Source: CAD feature listing. Evaluate the final solid. Frame: model axes, mm. Face numbers are marked on the shaded views. A direction names the side the tool comes from. Give positions to 0.01 mm unless a question says otherwise; leave off trailing zeros. Write each loop counter-clockwise with the first axis right and the second up, starting at its lowest first coordinate (ties: lowest second). Pieces come first, ordered by that corner, then holes. Notation, with made-up numbers: (-36.75, 29) -> (-6.75, 29) arc R18 cw to (-6.75, 54) -> close; hole circle Ø4 at (5.25, 21.5). An arc over 180 degrees is marked (long way). Write item = value, one per line.
from build123d import *

# Parameters (mm, degrees)
BOSS_EXTRUDE1_DEPTH = 2
BOSS_EXTRUDE2_DEPTH = 5
BOSS_EXTRUDE3_DEPTH = 1.5
FILLET1_R           = 2
CUT_EXTRUDE1_DEPTH  = 0.5


with BuildPart() as part:
    # Sketch1 → Boss-Extrude1 (new body)
    with BuildSketch(Plane(origin=(0, 0, 0), x_dir=(1, 0, 0), z_dir=(0, 1, 0))):
        with BuildLine():
            Line((-7.75, -13.25), (7.75, -13.25))
            ThreePointArc((7.75, -13.25), (9.871320344, -12.371320344), (10.75, -10.25))
            Line((10.75, -10.25), (10.75, 10.25))
            ThreePointArc((10.75, 10.25), (9.871320344, 12.371320344), (7.75, 13.25))
            Line((7.75, 13.25), (-7.75, 13.25))
            ThreePointArc((-7.75, 13.25), (-9.871320344, 12.371320344), (-10.75, 10.25))
            Line((-10.75, 10.25), (-10.75, -10.25))
            ThreePointArc((-10.75, -10.25), (-9.871320344, -12.371320344), (-7.75, -13.25))
        make_face()
    extrude(amount=BOSS_EXTRUDE1_DEPTH)

    # Sketch2 → Boss-Extrude2 (add)
    with BuildSketch(Plane(origin=(0, 2, 0), x_dir=(1, 0, 0), z_dir=(0, 1, 0))):
        with BuildLine():
            Line((-7.75, -13.25), (7.75, -13.25))
            ThreePointArc((7.75, -13.25), (9.871320344, -12.371320344), (10.75, -10.25))
            Line((10.75, -10.25), (10.75, 10.25))
            ThreePointArc((10.75, 10.25), (9.871320344, 12.371320344), (7.75, 13.25))
            Line((7.75, 13.25), (-7.75, 13.25))
            ThreePointArc((-7.75, 13.25), (-9.871320344, 12.371320344), (-10.75, 10.25))
            Line((-10.75, 10.25), (-10.75, -10.25))
            ThreePointArc((-10.75, -10.25), (-9.871320344, -12.371320344), (-7.75, -13.25))
        make_face()
        with BuildLine():
            Line((-7.75, -11.5), (7.75, -11.5))
            ThreePointArc((7.75, -11.5), (8.633883476, -11.133883476), (9, -10.25))
            Line((9, -10.25), (9, 10.25))
            ThreePointArc((9, 10.25), (8.633883476, 11.133883476), (7.75, 11.5))
            Line((7.75, 11.5), (-7.75, 11.5))
            ThreePointArc((-7.75, 11.5), (-8.633883476, 11.133883476), (-9, 10.25))
            Line((-9, 10.25), (-9, -10.25))
            ThreePointArc((-9, -10.25), (-8.633883476, -11.133883476), (-7.75, -11.5))
        make_face(mode=Mode.SUBTRACT)
    extrude(amount=BOSS_EXTRUDE2_DEPTH)

    # Sketch3 → Boss-Extrude3 (add)
    with BuildSketch(Plane(origin=(0, 2, 0), x_dir=(1, 0, 0), z_dir=(0, 1, 0))):
        with BuildLine():
            Line((9, -10.25), (-5.75, -10.25))
            ThreePointArc((-5.75, -10.25), (-7.164213562, -9.664213562), (-7.75, -8.25))
            Line((-7.75, -8.25), (-7.75, 8.25))
            ThreePointArc((-7.75, 8.25), (-7.164213562, 9.664213562), (-5.75, 10.25))
            Line((-5.75, 10.25), (9, 10.25))
            Line((9, 10.25), (9, 12.25))
            Line((9, 12.25), (-9.75, 12.25))
            Line((-9.75, 12.25), (-9.75, -12.25))
            Line((-9.75, -12.25), (9, -12.25))
            Line((9, -12.25), (9, -10.25))
        make_face()
    extrude(amount=BOSS_EXTRUDE3_DEPTH)

    # Fillet1
    fillet1_edges = [part.edges().sort_by_distance(p)[0] for p in [
        (0, 0, 13.25),
        (-9.871320344, 0, 12.371320344),
        (-10.75, 0, 0),
        (-9.871320344, 0, -12.371320344),
        (0, 0, -13.25),
        (9.871320344, 0, -12.371320344),
        (10.75, 0, 0),
        (9.871320344, 0, 12.371320344),
    ]]
    fillet(fillet1_edges, radius=FILLET1_R)

    # Sketch4 → Cut-Extrude1 (cut)
    with BuildSketch(Plane(origin=(0, 7, 0), x_dir=(1, 0, 0), z_dir=(0, 1, 0))):
        with BuildLine():
            Line((-7.75, 12.375), (7.75, 12.375))
            ThreePointArc((7.75, 12.375), (9.25260191, 11.75260191), (9.875, 10.25))
            Line((9.875, 10.25), (9.875, -10.25))
            ThreePointArc((9.875, -10.25), (9.25260191, -11.75260191), (7.75, -12.375))
            Line((7.75, -12.375), (-7.75, -12.375))
            ThreePointArc((-7.75, -12.375), (-9.25260191, -11.75260191), (-9.875, -10.25))
            Line((-9.875, -10.25), (-9.875, 10.25))
            ThreePointArc((-9.875, 10.25), (-9.25260191, 11.75260191), (-7.75, 12.375))
        make_face()
    extrude(amount=-CUT_EXTRUDE1_DEPTH, mode=Mode.SUBTRACT)


solid = part.part
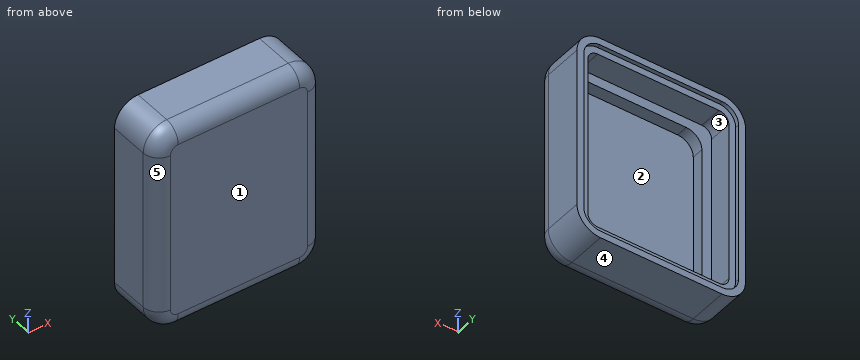
(1) Section query B-B (z = -3). Return loops of the section in (x, y) (3 decimals), plus the area to 3 significant figures.
Values follow:
outline = (-10.75, 2) arc R2 ccw to (-8.75, 0) -> (8.75, 0) arc R2 ccw to (10.75, 2) -> (10.75, 7) -> (9.875, 7) -> (9.875, 6.5) -> (9, 6.5) -> (9, 2) -> (-7.75, 2) -> (-7.75, 3.5) -> (-9, 3.5) -> (-9, 6.5) -> (-9.875, 6.5) -> (-9.875, 7) -> (-10.75, 7) -> close
area = 59.8 mm2
(2) Section query D-D (y = 3). Return loops of the section in (x, z).
Values follow:
outline = (-10.75, -10.25) arc R3 ccw to (-7.75, -13.25) -> (7.75, -13.25) arc R3 ccw to (10.75, -10.25) -> (10.75, 10.25) arc R3 ccw to (7.75, 13.25) -> (-7.75, 13.25) arc R3 ccw to (-10.75, 10.25) -> close; hole (-7.75, -8.25) arc R2 ccw to (-5.75, -10.25) -> (9, -10.25) -> (9, 10.25) -> (-5.75, 10.25) arc R2 ccw to (-7.75, 8.25) -> close
(3) Pull-direction query (X, two-part tool) for the marked faces 3, 4 and 5; classes: pulls with the +X half, pulls with the -X half, needs draft (parallel to the pull), parting line crosses it, or undercut.
Values follow:
face_3 = undercut
face_4 = needs draft
face_5 = pulls with the -X half
(4) Access query for the marked faces 1 and 2. Directions: +Z, -Z, +X, -X, +Y, -Y. A direction counts if a zero-diameter tool reaches every point of the face in a straight line with its end or side. Return the directions, or none.
Values follow:
face_1 = +Z, -Z, +X, -X, -Y
face_2 = +Y
(5) Section query A-A (y = 5.5). Return loops of the section in (x, z).
Values follow:
outline = (-10.75, -10.25) arc R3 ccw to (-7.75, -13.25) -> (7.75, -13.25) arc R3 ccw to (10.75, -10.25) -> (10.75, 10.25) arc R3 ccw to (7.75, 13.25) -> (-7.75, 13.25) arc R3 ccw to (-10.75, 10.25) -> close; hole (-9, -10.25) arc R1.25 ccw to (-7.75, -11.5) -> (7.75, -11.5) arc R1.25 ccw to (9, -10.25) -> (9, 10.25) arc R1.25 ccw to (7.75, 11.5) -> (-7.75, 11.5) arc R1.25 ccw to (-9, 10.25) -> close
(6) First-contact query: pin 1 (12 mm diameter, centred on x = 0.5, z = 9.5, fed in from +Y); pin 2 (6 mm diameter, centred on x = 1.5, z = 0.5, fed in from +Y). Flat tips, straight axial feed; report the tip coordinate or a pass-through.
Values follow:
pin_1 = 7
pin_2 = 2
(7) Section query C-C (x = 6.75). Return loops of the section in (y, z) (3 decimals), plus the area to 3 significant figures.
Values follow:
outline = (0, -11.25) arc R2 ccw to (2, -13.25) -> (7, -13.25) -> (7, -12.375) -> (6.5, -12.375) -> (6.5, -11.5) -> (3.5, -11.5) -> (3.5, -10.25) -> (2, -10.25) -> (2, 10.25) -> (3.5, 10.25) -> (3.5, 11.5) -> (6.5, 11.5) -> (6.5, 12.375) -> (7, 12.375) -> (7, 13.25) -> (2, 13.25) arc R2 ccw to (0, 11.25) -> close
area = 71.7 mm2
(8) Material intervals for line 1 (X direction, y = 5.75, z = 10.25); line 2 (Z direction, x = -1, y = 6); line 3 (Z direction, x = 4.5, y = 6.75) (3 decimals), sorted ascending.
Values follow:
line_1 = -10.75 to -9, 9 to 10.75
line_2 = -13.25 to -11.5, 11.5 to 13.25
line_3 = -13.25 to -12.375, 12.375 to 13.25
